```python
from build123d import *

# Parameters (mm, degrees)
F1_DEPTH    = 5
F2_T1_DEPTH = 6.2718359258
F2_T3_DEPTH = 6.2718359258
F3_R        = 2.6
F4_DEPTH    = 27.001
F5_SIZE     = 0.5


# Not quite as in the source:
# - a fillet or chamfer that OpenCascade refuses, or shapes differently, is made with other operations: its cross-section is extruded or revolved along the edge and cut away or added
# - a pattern or mirror of a feature is missing from the dataset's text; its kind, count and spacing are read off the source's solid


with BuildPart() as f1:
    # F0 (on Front) → F1 (new body, symmetric)
    with BuildSketch(Plane.XZ):
        with BuildLine():
            ThreePointArc((0, 20), (13.7840487521, 14.4913767462), (19.9749843554, 1))
            Line((19.9749843554, 1), (29, 1))
            Line((29, 1), (29, 28))
            Line((29, 28), (19, 28))
            Line((19, 28), (19, 18.3303027798))
            ThreePointArc((19, 18.3303027798), (17.8, 16.4972725018), (15.64, 16.8638785574))
            ThreePointArc((15.64, 16.8638785574), (8.4003212194, 21.4110859933), (0, 23))
            ThreePointArc((0, 23), (-8.4003212194, 21.4110859933), (-15.64, 16.8638785574))
            ThreePointArc((-15.64, 16.8638785574), (-17.8, 16.4972725018), (-19, 18.3303027798))
            Line((-19, 18.3303027798), (-19, 28))
            Line((-19, 28), (-29, 28))
            Line((-29, 28), (-29, 1))
            Line((-29, 1), (-19.9749843554, 1))
            ThreePointArc((-19.9749843554, 1), (-13.7840487521, 14.4913767462), (0, 20))
        make_face()
    extrude(amount=F1_DEPTH, both=True)

    # F2: chamfer of 0.5 on 4 edges, made by hand

    # F2_s2 → F2_t1 (cut)
    with BuildSketch(Plane.XZ.offset(-6.2718359258)):
        with BuildLine():
            Line((19.9300167465, 1.500192138), (20.4835367376, 0.9863935992))
            Line((20.4835367376, 0.9863935992), (20.4835367376, 0.9763935992))
            ThreePointArc((20.4835367376, 0.9763935992), (20.2292605465, 0.99), (19.9749843554, 0.99))
            Line((19.9749843554, 0.99), (19.9649968633, 0.9995))
            ThreePointArc((19.9649968633, 0.9995), (19.9508800221, 1.249994537), (19.920044409, 1.4994488451))
            Line((19.920044409, 1.4994488451), (19.9300167465, 1.500192138))
        make_face()
        with BuildLine():
            Line((-19.9300167465, 1.500192138), (-20.4835367376, 0.9863935992))
            Line((-20.4835367376, 0.9863935992), (-20.4835367376, 0.9763935992))
            ThreePointArc((-20.4835367376, 0.9763935992), (-20.2292605465, 0.99), (-19.9749843554, 0.99))
            Line((-19.9749843554, 0.99), (-19.9649968633, 0.9995))
            ThreePointArc((-19.9649968633, 0.9995), (-19.9508800221, 1.249994537), (-19.920044409, 1.4994488451))
            Line((-19.920044409, 1.4994488451), (-19.9300167465, 1.500192138))
        make_face()
    extrude(amount=F2_T1_DEPTH, mode=Mode.SUBTRACT)

    # F2_s4 → F2_t3 (cut)
    with BuildSketch(Plane.XZ):
        with BuildLine():
            Line((19.9300167465, 1.500192138), (20.4835367376, 0.9863935992))
            Line((20.4835367376, 0.9863935992), (20.4835367376, 0.9763935992))
            ThreePointArc((20.4835367376, 0.9763935992), (20.2292605465, 0.99), (19.9749843554, 0.99))
            Line((19.9749843554, 0.99), (19.9649968633, 0.9995))
            ThreePointArc((19.9649968633, 0.9995), (19.9508800221, 1.249994537), (19.920044409, 1.4994488451))
            Line((19.920044409, 1.4994488451), (19.9300167465, 1.500192138))
        make_face()
        with BuildLine():
            Line((-19.9300167465, 1.500192138), (-20.4835367376, 0.9863935992))
            Line((-20.4835367376, 0.9863935992), (-20.4835367376, 0.9763935992))
            ThreePointArc((-20.4835367376, 0.9763935992), (-20.2292605465, 0.99), (-19.9749843554, 0.99))
            Line((-19.9749843554, 0.99), (-19.9649968633, 0.9995))
            ThreePointArc((-19.9649968633, 0.9995), (-19.9508800221, 1.249994537), (-19.920044409, 1.4994488451))
            Line((-19.920044409, 1.4994488451), (-19.9300167465, 1.500192138))
        make_face()
    extrude(amount=F2_T3_DEPTH, mode=Mode.SUBTRACT)

    # F3 (on face) → F4 (cut, through all)
    with BuildSketch(Plane.XY.offset(28)):
        with Locations((24, 0)):
            Circle(F3_R)
    f4 = extrude(amount=-F4_DEPTH, mode=Mode.SUBTRACT)

    # F4_copies: F4 across plane
    add(f4.mirror(Plane(origin=(0, 0, 0), x_dir=(0, 0, -1), z_dir=(-1, 0, 0))), mode=Mode.SUBTRACT)

    # F5
    f5_edges = [f1.edges().sort_by_distance(p)[0] for p in [
        (24, 2.6, 28),
        (24, -2.6, 28),
        (24, 2.6, 1),
        (-24, 2.6, 1),
        (-24, 2.6, 28),
        (24, -2.6, 1),
        (-24, -2.6, 1),
        (-24, -2.6, 28),
    ]]
    chamfer(f5_edges, length=F5_SIZE)


solid = f1.part
```
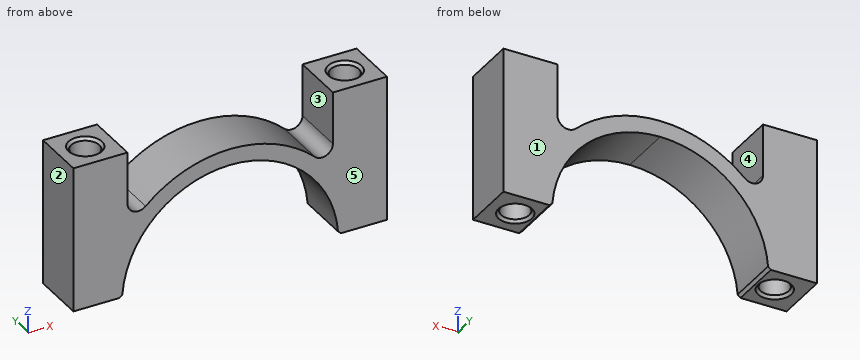
CAD build for the part. Positions are in the model's coordinates, mm. Face numbers are marked on the shaded views. A direction names the side the tool comes from. Round coordinates to 2 decimals unless told otherwise and drop trailing zeros. Order: outer loops, then holes, each group sorted by start corner. A loop starts at its lowest first (then second) coordinate and runs counter-clockwise, first axis right, second up. Notation, with made-up numbers: (11.5, -5) - (15.5, -5) arc R38 cw to (15.5, 33) - close; hole circle Ø9 at (-5, -7.75). An arc over 180 degrees is marked (long way). Answer in a Markdown table with one row per item. Add a question column.
(1) Band-saw the part on C-C on x = -24. List the corners of the cut face in (y, z), and give its area (3 significant figures).
(2) Band-saw the part on D-D on z = 20.75. List the corners of the cut face in (x, y).
(3) Mould opens along X. For the marked faces 1, 2 and 3 say: +X half, -X half, draft (parallel to the pull), parting line (faces both ways), or undercut.
(4) Band-saw the part on B-B on y = 0. Count the separate pieces of the cut face and the enclosed holes in it, and give its area (3 significant figures).
(5) Band-saw the part on A-A on z = 12. List the corners of the cut face in (x, y), and give its area (3 significant figures).
(6) 3-axis set-ups, long thin cutter, end or side, ignore diameter. For the marked faces 4 and 5: which of +Z, -Z, +X, -X, +Y, -Y reach the whole face in a straight line?
(7) Drop flat-ended pins along their axis: pin 1 Ø1.5 at (x, y) = (-12.5, 0) entering from -Z; pin 2 Ø2 at (x, y) = (13, 3.5) entering from -Z; pin 3 Ø4 at (x, y) = (3.5, 3) entering from -Z. Give the stop position or say it passes through.
(8) Probe L1, parallel to Y at x = 24, z = 20.75; L2, parallel to X at y = 2.25, z = 23.5; L3, parallel to X at y = -4, z = 17.5. List the from-to ranges inside material, lowest first. Write a range as [from, to].
Data:
| question | item | result |
|---|---|---|
| 1 | outline | (-5, 1) - (-3.1, 1) - (-2.6, 1.5) - (-2.6, 27.5) - (-3.1, 28) - (-5, 28) - close; (2.6, 1.5) - (3.1, 1) - (5, 1) - (5, 28) - (3.1, 28) - (2.6, 27.5) - close |
| 1 | area | 129 mm^2 |
| 2 | outline | (-29, -5) - (-19, -5) - (-19, 5) - (-29, 5) - close; (-9.92, -5) - (9.92, -5) - (9.92, 5) - (-9.92, 5) - close; (19, -5) - (29, -5) - (29, 5) - (19, 5) - close; hole circle Ø5.2 at (-24, 0); hole circle Ø5.2 at (24, 0) |
| 3 | face 1 | draft |
| 3 | face 2 | -X half |
| 3 | face 3 | undercut |
| 4 | separate pieces | 3 |
| 4 | enclosed holes | 0 |
| 4 | area | 403 mm^2 |
| 5 | outline | (-29, -5) - (-16, -5) - (-16, 5) - (-29, 5) - close; (16, -5) - (29, -5) - (29, 5) - (16, 5) - close; hole circle Ø5.2 at (-24, 0); hole circle Ø5.2 at (24, 0) |
| 5 | area | 218 mm^2 |
| 6 | face 4 | +Z, +Y, -Y |
| 6 | face 5 | +Z, -Z, +X, -X, -Y |
| 7 | pin 1 | stops at z = 14.98 |
| 7 | pin 2 | stops at z = 14.28 |
| 7 | pin 3 | stops at z = 19.23 |
| 8 | L1 | y = [-5, -2.6], [2.6, 5] |
| 8 | L2 | x = [-29, -25.3], [-22.7, -19], [19, 22.7], [25.3, 29] |
| 8 | L3 | x = [-29, -18.82], [-14.92, -9.68], [9.68, 14.92], [18.82, 29] |
